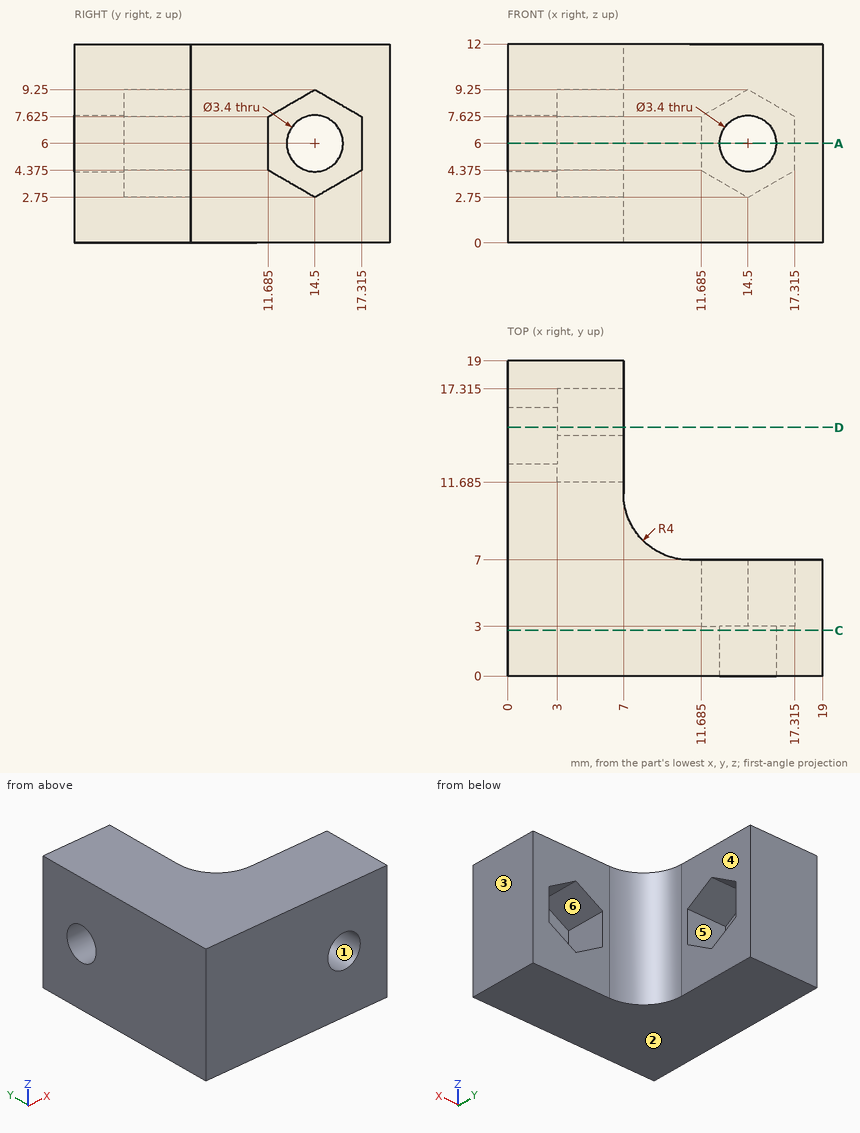
Geometry: see drawing. Coordinates: mm, zero at the bounding-box minimum. A direction names the side the tool comes from. Coordinates: 2 decimals unless noted, no trailing zeros. Loops run counter-clockwise (first coordinate to the right, second up) from the corner with the lowest first, then second, coordinate; pieces in that order, holes last. Notation, with made-up numbers: (76, -30) -> (80, -30) arc R9 cw to (80, -17) -> close; hole circle Ø1 at (30.5, -28). An arc over 180 degrees is marked (long way). Use a Markdown table: item, result.
1) Access query for the marked faces 4, 5 and 6. Directions: +Z, -Z, +X, -X, +Y, -Y. A direction counts if a zero-diameter tool reaches every point of the face in a straight line with its end or side. Return the directions, or none.
Results found:
| item | result |
|---|---|
| face 4 | +Z, -Z, +X, +Y |
| face 5 | +X |
| face 6 | +Y |
2) Contact query for flat-ended pins moving along their axis: pin 1 (3 mm diameter, centred on y = 15, z = 6.5, fed in from +X); pin 2 (2 mm diameter, centred on y = 10.5, z = 6, fed in from +X); pin 3 (6 mm diameter, centred on y = 9, z = 1.5, fed in from +X); pin 4 (8 mm diameter, centred on x = 12.5, y = 11.5, fed in from -Z). Output: stop coordinate, or through.
Results found:
| item | result |
|---|---|
| pin 1 | stops at x = 3 |
| pin 2 | stops at x = 7.29 |
| pin 3 | stops at x = 19 |
| pin 4 | passes through |
3) Pull-direction query (Z, two-part tool) for the marked faces 1, 2 and 3; classes: released by +Z, released by -Z, zero draft, split by the parting line, or undercut.
Results found:
| item | result |
|---|---|
| face 1 | undercut |
| face 2 | released by -Z |
| face 3 | zero draft |
4) Cut plane D-D (y = 15). Return the cut outline in (x, z) (1 decimal).
Results found:
| item | result |
|---|---|
| outline | (0, 0) -> (7, 0) -> (7, 3) -> (3, 3) -> (3, 4.4) -> (0, 4.4) -> close; (0, 7.6) -> (3, 7.6) -> (3, 9) -> (7, 9) -> (7, 12) -> (0, 12) -> close |
5) Cut plane C-C (y = 2.75). Return the cut outline in (x, z), then the cut area to 3 significant figures.
Results found:
| item | result |
|---|---|
| outline | (0, 0) -> (19, 0) -> (19, 12) -> (0, 12) -> close; hole circle Ø3.4 at (14.5, 6) |
| area | 219 mm2 |
6) Cut plane A-A (z = 6). Return the cut outline in (x, y) (1 decimal).
Results found:
| item | result |
|---|---|
| outline | (0, 0) -> (12.8, 0) -> (12.8, 3) -> (11.7, 3) -> (11.7, 7) -> (11, 7) arc R4 cw to (7, 11) -> (7, 11.7) -> (3, 11.7) -> (3, 12.8) -> (0, 12.8) -> close; (0, 16.2) -> (3, 16.2) -> (3, 17.3) -> (7, 17.3) -> (7, 19) -> (0, 19) -> close; (16.2, 0) -> (19, 0) -> (19, 7) -> (17.3, 7) -> (17.3, 3) -> (16.2, 3) -> close |
7) Material intervals for line 1 along X through (y, z) = (2.1, 6); line 2 along Z through (x, y) = (14.5, 0.85), sorted ascending. Write a range as from..to.
Results found:
| item | result |
|---|---|
| line 1 | x = 0..12.8, 16.2..19 |
| line 2 | z = 0..4.3, 7.7..12 |
